Part print with two shaded views. Sizes in mm from the minimum x, y, z corner. Round coordinates to 2 decimals unless told otherwise and drop trailing zeros. Loops run counter-clockwise (first coordinate to the right, second up) from the corner with the lowest first, then second, coordinate; pieces in that order, holes last.
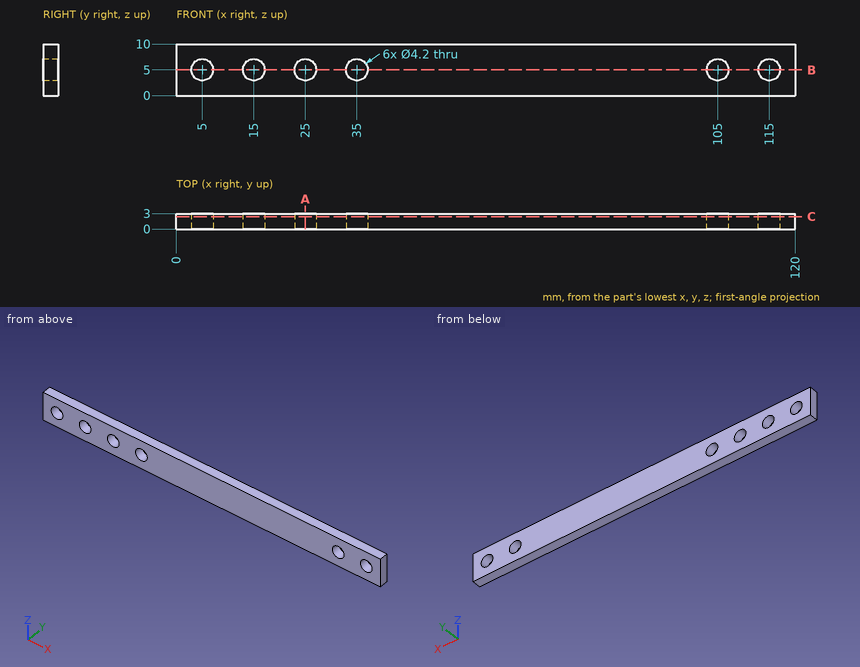
Item 1: Flat gauge pins, fed straight in: P1, Ø1.5, axis at y = 2.5, z = 3.5, coming from the -X side; P2, Ø2.5, axis at x = 25, z = 5, coming from the -Y side. Where does each tip first touch, or does it go through?
Verdict:
P1: stops at x = 0
P2: passes through
Item 2: Cut at C-C (y = 2.4). List the corners of the cut face in (x, z), plus the area to 3 significant figures.
Verdict:
outline: (0, 0) - (120, 0) - (120, 10) - (0, 10) - close; hole circle Ø4.2 at (5, 5); hole circle Ø4.2 at (15, 5); hole circle Ø4.2 at (25, 5); hole circle Ø4.2 at (35, 5); hole circle Ø4.2 at (105, 5); hole circle Ø4.2 at (115, 5)
area: 1,120 mm2
Item 3: Wall check: L1, parallel to Z at x = 105, y = 2.35; L2, parallel to Z at x = 114, y = 0.5. Give the ranges that are in metal, low to high.
Verdict:
L1: z = 0 to 2.9, 7.1 to 10
L2: z = 0 to 3.15, 6.85 to 10
Item 4: Cut at A-A (x = 25). List the corners of the cut face in (y, z).
Verdict:
outline: (0, 0) - (3, 0) - (3, 2.9) - (0, 2.9) - close; (0, 7.1) - (3, 7.1) - (3, 10) - (0, 10) - close
Item 5: Cut at B-B (z = 5). List the corners of the cut face in (x, y), plus the area to 3 significant figures.
Verdict:
outline: (0, 0) - (2.9, 0) - (2.9, 3) - (0, 3) - close; (7.1, 0) - (12.9, 0) - (12.9, 3) - (7.1, 3) - close; (17.1, 0) - (22.9, 0) - (22.9, 3) - (17.1, 3) - close; (27.1, 0) - (32.9, 0) - (32.9, 3) - (27.1, 3) - close; (37.1, 0) - (102.9, 0) - (102.9, 3) - (37.1, 3) - close; (107.1, 0) - (112.9, 0) - (112.9, 3) - (107.1, 3) - close; (117.1, 0) - (120, 0) - (120, 3) - (117.1, 3) - close
area: 284 mm2
